from build123d import *

# Parameters (mm, degrees)
SKETCH1_R               = 87
SKETCH1_R_2             = 85
BOSS_EXTRUDE1_DEPTH     = 225
CUT_EXTRUDE1_REACH      = 299.439
CUT_EXTRUDE1_END_RADIUS = 85
SKETCH2_R               = 2
CIRPATTERN1_COUNT       = 6


with BuildPart() as part:
    # Sketch1 → Boss-Extrude1 (new body)
    with BuildSketch(Plane(origin=(0, 0, 0), x_dir=(1, 0, 0), z_dir=(0, 1, 0))):
        with Locations(Location((0, 0, 0), (0, 0, 270))):
            Circle(SKETCH1_R)
        with Locations(Location((0, 0, 0), (0, 0, 270))):
            Circle(SKETCH1_R_2, mode=Mode.SUBTRACT)
    extrude(amount=BOSS_EXTRUDE1_DEPTH)

    # Cut-Extrude1: up to this cylinder (the profile starts outside it)
    cut_extrude1_end = Plane(origin=(0, 7.5, 0), z_dir=(0, -1, 0)) * Cylinder(CUT_EXTRUDE1_END_RADIUS, 769.878, mode=Mode.PRIVATE)
    # Sketch2 → Cut-Extrude1 (cut, up to the surface)
    with BuildSketch(Plane.ZY.offset(87), mode=Mode.PRIVATE) as cut_extrude1_sk1:
        with Locations((0, 7.5)):
            Circle(SKETCH2_R)
    cut_extrude1_tool1 = extrude(cut_extrude1_sk1.sketch, amount=-CUT_EXTRUDE1_REACH, mode=Mode.PRIVATE) - cut_extrude1_end
    cut_extrude1 = cut_extrude1_tool1.solids().sort_by_distance((-87, 7.5, 0))[0]
    add(cut_extrude1, mode=Mode.SUBTRACT)

    # CirPattern1: Cut-Extrude1 ×6 about axis
    cirpattern1_axis = Axis((0, 0, 0), (0, 1, 0))
    for i in range(1, CIRPATTERN1_COUNT):
        add(cut_extrude1.rotate(cirpattern1_axis, i * 360 / CIRPATTERN1_COUNT), mode=Mode.SUBTRACT)


solid = part.part
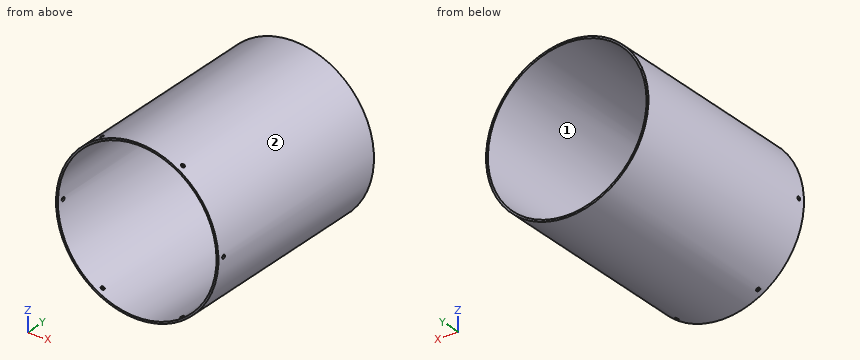
Here's how the part is built. I have some questions about the finished solid (model axes, mm). Face numbers are marked on the shaded views. Coordinates: 2 decimals unless noted, no trailing zeros. Order: outer loops, then holes, each group sorted by start corner. A loop starts at its lowest first (then second) coordinate and runs counter-clockwise, first axis right, second up. Notation, with made-up numbers: M 70,9.25 L 121,9.25 A13 cw 121,33.25 Z; hole C 80,5.5 d3. An arc over 180 degrees is marked long. Answer as CSV lines item,"result". Start each with the question number.
1. I want a section at A-A, the plane x = 0. Write out the boundary of the cut face in (y, z), and give its area (3 significant figures).
2. We'd pull the mould along Z, two halves only. Please class the marked faces 1 and 2: released by +Z, released by -Z, zero draft, split by the parting line, or undercut.
3. I want a section at C-C, the plane y = 20.5. Write out the boundary of the cut face in (x, z), and give its area (3 significant figures).
4. For pin 1 (10 mm diameter, centred on x = -5.5, y = 76, fed in from +Z); pin 2 (1 mm diameter, centred on x = -41, y = 154, fed in from +Z); pin 3 (10 mm diameter, centred on x = 38, z = 69.5, fed in from -Y); pin 4 (4 mm diameter, centred on x = 33, y = 27.5, fed in from +Z), each with a flat end and sliding along its axis, tell me the tip position at first contact or that it passes through.
5. I need wall thicknesses on line 1 (X direction, y = 82.5, z = 0); line 2 (Y direction, x = 86, z = 0); line 3 (X direction, y = 43, z = -12). Which ranges of each line are inside material? Lowest first, please. Write a range as [from, to].
6. I want a section at B-B, the plane z = 7.5. Write out the boundary of the cut face in (x, y).
Recorded:
1,outline,"M 0,-87 L 225,-87 L 225,-85 L 0,-85 Z; M 0,85 L 225,85 L 225,87 L 0,87 Z"
1,area,"900 mm2"
2,face 1,"undercut"
2,face 2,"split by the parting line"
3,outline,"C 0,0 d174; hole C 0,0 d170"
3,area,"1,080 mm2"
4,pin 1,"stops at z = 87"
4,pin 2,"stops at z = 77"
4,pin 3,"passes through"
4,pin 4,"stops at z = 81.29"
5,line 1,"x = [-87, -85], [85, 87]"
5,line 2,"y = [0, 5.5], [9.5, 225]"
5,line 3,"x = [-86.17, -84.15], [84.15, 86.17]"
6,outline,"M -86.68,0 L -84.67,0 L -84.67,225 L -86.68,225 Z; M 84.67,0 L 86.68,0 L 86.68,225 L 84.67,225 Z"
